from build123d import *

# Parameters (mm, degrees)
SKETCH_W        = 75
SKETCH_H        = 56
PAD_DEPTH       = 15
SKETCH001_R     = 6
POCKET_DEPTH    = 15.001
SKETCH002_W     = 111.933372
SKETCH002_H     = 32
POCKET001_DEPTH = 5
PAD001_DEPTH    = 6
SKETCH004_R     = 18
PAD002_DEPTH    = 25
SKETCH005_R     = 11
POCKET002_DEPTH = 63.001


with BuildPart() as pocket001:
    # Sketch → Pad (new body)
    with BuildSketch(Plane.XY):
        Rectangle(SKETCH_W, SKETCH_H)
    extrude(amount=PAD_DEPTH)

    # Sketch001 → Pocket (cut, through all)
    with BuildSketch(Plane.XY.offset(15)):
        with Locations((-22.5, 0)):
            Circle(SKETCH001_R)
        with Locations((22.5, 0)):
            Circle(SKETCH001_R)
    extrude(amount=-POCKET_DEPTH, mode=Mode.SUBTRACT)

    # Sketch002 → Pocket001 (cut)
    with BuildSketch(Plane(origin=(0, 0, 0), x_dir=(1, 0, 0), z_dir=(0, 0, -1))):
        with Locations((5.213337, 0)):
            Rectangle(SKETCH002_W, SKETCH002_H)
    extrude(amount=-POCKET001_DEPTH, mode=Mode.SUBTRACT)


with BuildPart() as fusion:
    # Sketch003 → Pad001 (new body, symmetric)
    with BuildSketch(Plane.YZ):
        Polygon((-28, 0), (28, 0), (54, 38), (54, 63), (36, 63), (-28, 15), align=None)
    extrude(amount=PAD001_DEPTH, both=True)

    # Sketch004 → Pad002 (new body)
    with BuildSketch(Plane(origin=(0, 0, 63), x_dir=(0, -1, 0), z_dir=(0, 0, 1))):
        with Locations((-70.970563, 0)):
            Circle(SKETCH004_R)
    extrude(amount=-PAD002_DEPTH)

    # Sketch005 → Pocket002 (cut, through all)
    with BuildSketch(Plane(origin=(0, 0, 63), x_dir=(0, -1, 0), z_dir=(0, 0, 1))):
        with Locations((-70.970563, 0)):
            Circle(SKETCH005_R)
    extrude(amount=-POCKET002_DEPTH, mode=Mode.SUBTRACT)

    # Fusion: union Pocket001
    add(pocket001.part)


solid = fusion.part
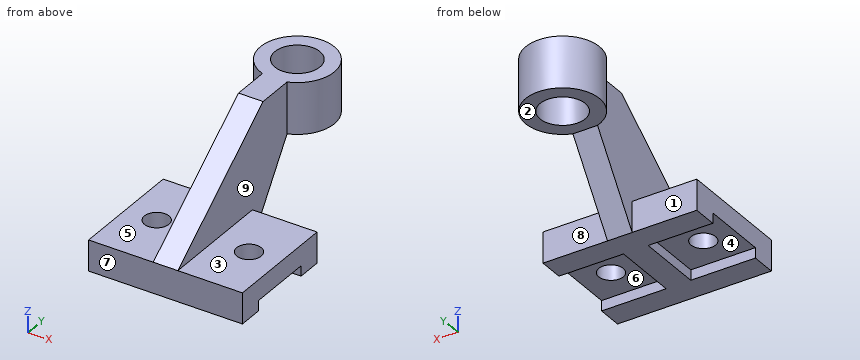
Read the model definition and answer for the solid it produces. Units are mm, in the model's axes. Face numbers are marked on the shaded views. A direction names the side the tool comes from. Give positions to 0.01 mm unless a question says otherwise; leave off trailing zeros. Write each loop counter-clockwise with the first axis right and the second up, starting at its lowest first coordinate (ties: lowest second). Pieces come first, ordered by that corner, then holes. Notation, with made-up numbers: (2, 41) - (8, 41) arc R14 ccw to (8, 64) - close; hole circle Ø7 at (88.25, 84.5). An arc over 180 degrees is marked (long way). Answer in a Markdown table with one row per item. Add a question column.
Item 1: Section A-A, the plane x = 0 is taken. Write down the section's boundary in (y, z), and give its area (3 significant figures).
Item 2: Section B-B, the plane y = 0 is taken. Write down the section's boundary in (x, z).
Item 3: Section D-D, the plane y = 80.5 is taken. Write down the section's boundary in (x, z).
Item 4: Section C-C, the plane x = 31 is taken. Write down the section's boundary in (y, z), and give its area (3 significant figures).
Item 5: Find the intervals of material crossed by L1, parallel to Y at x = 22, z = 13; L2, parallel to Y at x = 14, z = 3.5; L3, parallel to Z at x = 11, y = 22, in increasing order.
Item 6: Determine the mould class of the marked faces 6, 7, 8 and 9 for opening direction Y: pulls with the +Y half, pulls with the -Y half, needs draft (parallel to the pull), parting line crosses it, or undercut.
Item 7: Flat-ended cylindrical pins translate along their axes: P1, Ø1, axis at x = 3.5, z = 26.5, coming from the -Y side; P2, Ø1.5, axis at y = 5.5, z = 2.5, coming from the +X side; P3, Ø12, axis at y = 24.5, z = 19, coming from the +X side; P4, Ø1, axis at x = 5, z = 11.5, coming from the +Y side. Find the tip coordinate at first contact, or state that the pin passes through.
Item 8: A tool of negligible diameter and unlimited length cuts with its end or side. For the marked faces 1, 2, 3, 4 and 5, from which of +Z, -Z, +X, -X, +Y, -Y can it reach the whole face along a straight path? Write none if from no direction.
Recorded:
| question | item | result |
|---|---|---|
| 1 | outline | (-28, 0) - (28, 0) - (54, 38) - (59.97, 38) - (59.97, 63) - (36, 63) - (-28, 15) - close; (81.97, 38) - (88.97, 38) - (88.97, 63) - (81.97, 63) - close |
| 1 | area | 3,460 mm2 |
| 2 | outline | (-37.5, 5) - (-28.5, 5) - (-28.5, 15) - (-37.5, 15) - close; (-16.5, 5) - (-6, 5) - (-6, 0) - (6, 0) - (6, 5) - (16.5, 5) - (16.5, 15) - (6, 15) - (6, 36) - (-6, 36) - (-6, 15) - (-16.5, 15) - close; (28.5, 5) - (37.5, 5) - (37.5, 15) - (28.5, 15) - close |
| 3 | outline | (-15.27, 38) - (-5.49, 38) - (-5.49, 63) - (-15.27, 63) - close; (5.49, 38) - (15.27, 38) - (15.27, 63) - (5.49, 63) - close |
| 4 | outline | (-28, 0) - (-16, 0) - (-16, 5) - (16, 5) - (16, 0) - (28, 0) - (28, 15) - (-28, 15) - close |
| 4 | area | 680 mm2 |
| 5 | L1 | y = -28 to -5.98, 5.98 to 28 |
| 5 | L2 | y = -28 to -16, 16 to 28 |
| 5 | L3 | z = 0 to 15 |
| 6 | face 6 | undercut |
| 6 | face 7 | pulls with the -Y half |
| 6 | face 8 | pulls with the +Y half |
| 6 | face 9 | needs draft |
| 7 | P1 | stops at y = -13.33 |
| 7 | P2 | stops at x = 6 |
| 7 | P3 | stops at x = 37.5 |
| 7 | P4 | stops at y = 36.21 |
| 8 | face 1 | +Z, -Z, -X, +Y |
| 8 | face 2 | -Z, +X, -X, +Y |
| 8 | face 3 | +Z, +X, +Y, -Y |
| 8 | face 4 | -Z, -X |
| 8 | face 5 | +Z, -X, +Y, -Y |
